Geometry: final body of the model. Coordinates: model frame, mm. A direction names the side the tool comes from. Round coordinates to 2 decimals unless told otherwise and drop trailing zeros. Write each loop counter-clockwise with the first axis right and the second up, starting at its lowest first coordinate (ties: lowest second). Pieces come first, ordered by that corner, then holes. Notation, with made-up numbers: (-30.75, -15) - (1.25, -15) arc R21 ccw to (1.25, 5) - close; hole circle Ø11 at (9.25, 38.25). An arc over 180 degrees is marked (long way). Use a Markdown table: item, result. Add a question column.
```python
from build123d import *

# Parameters (mm, degrees)
SKETCH1_W           = 37
SKETCH1_H           = 8
SKETCH1_R           = 1.75
BOSS_EXTRUDE1_DEPTH = 5
SKETCH2_W           = 4
SKETCH2_H           = 8
BOSS_EXTRUDE2_DEPTH = 12.5
SKETCH4_W           = 4
SKETCH4_H           = 7.5
BOSS_EXTRUDE3_DEPTH = 8
SKETCH3_R           = 1.75
CUT_EXTRUDE1_DEPTH  = 37.745748053
FILLET1_R           = 4
SKETCH6_R           = 1.6
BOSS_EXTRUDE5_DEPTH = 4


with BuildPart() as part:
    # Sketch1 → Boss-Extrude1 (new body)
    with BuildSketch(Plane.XY):
        Rectangle(SKETCH1_W, SKETCH1_H)
        with Locations((-15, 0)):
            Circle(SKETCH1_R, mode=Mode.SUBTRACT)
        with Locations(Location((15, 0, 0), (0, 0, 180))):
            Circle(SKETCH1_R, mode=Mode.SUBTRACT)
    extrude(amount=BOSS_EXTRUDE1_DEPTH)

    # Sketch2 → Boss-Extrude2 (add)
    with BuildSketch(Plane.XY.offset(5)):
        with Locations((-9.5, 0)):
            Rectangle(SKETCH2_W, SKETCH2_H)
        with Locations((9.5, 0)):
            Rectangle(SKETCH2_W, SKETCH2_H)
    extrude(amount=BOSS_EXTRUDE2_DEPTH)

    # Sketch4 → Boss-Extrude3 (add)
    with BuildSketch(Plane(origin=(0, 4, 0), x_dir=(1, 0, 0), z_dir=(0, 1, 0))):
        with Locations((-9.5, -13.75)):
            Rectangle(SKETCH4_W, SKETCH4_H)
        with Locations((9.5, -13.75)):
            Rectangle(SKETCH4_W, SKETCH4_H)
    extrude(amount=BOSS_EXTRUDE3_DEPTH)

    # Sketch3 → Cut-Extrude1 (cut, through all)
    with BuildSketch(Plane.ZY.offset(11.5)):
        with Locations(Location((13.75, 8.5, 0), (0, 0, 270))):
            Circle(SKETCH3_R)
    extrude(amount=-CUT_EXTRUDE1_DEPTH, mode=Mode.SUBTRACT)

    # Fillet1
    # the kernel refuses this fillet: 4 mm, written as the material it takes off along each edge
    with BuildSketch(Plane(origin=(2.5, 12, 10), x_dir=(0, -1, 0), z_dir=(-1, 0, 0))) as fillet1_piece_1:
        with BuildLine():
            CenterArc((FILLET1_R, FILLET1_R), FILLET1_R, 180, 90)
            Line((0, FILLET1_R), (0, 0))
            Line((0, 0), (FILLET1_R, 0))
        make_face()
    extrude(amount=24, mode=Mode.SUBTRACT)
    with BuildSketch(Plane(origin=(-2.5, 12, 10), x_dir=(0, -1, 0), z_dir=(1, 0, 0)), Plane(origin=(21.5, 12, 17.5), x_dir=(0, -1, 0), z_dir=(-1, 0, 0)), Plane(origin=(-21.5, 12, 17.5), x_dir=(0, 0, -1), z_dir=(1, 0, 0))) as fillet1_piece_2:
        with BuildLine():
            CenterArc((FILLET1_R, -FILLET1_R), FILLET1_R, 90, 90)
            Line((0, -FILLET1_R), (0, 0))
            Line((0, 0), (FILLET1_R, 0))
        make_face()
    extrude(amount=24, mode=Mode.SUBTRACT)

    # Sketch6 → Boss-Extrude5 (add)
    with BuildSketch(Plane.ZY.offset(11.5)):
        with BuildLine():
            Line((56.011251263, -29.401227517), (11.782401197, -4))
            Line((11.782401197, -4), (17.5, 1.941786969))
            Line((17.5, 1.941786969), (59.995440826, -22.463920148))
            ThreePointArc((59.995440826, -22.463920148), (61.471999729, -27.924668614), (56.011251263, -29.401227517))
        make_face()
        with Locations(Location((58.003346044, -25.932573832, 0), (0, 0, 270))):
            Circle(SKETCH6_R, mode=Mode.SUBTRACT)
    extrude(amount=-BOSS_EXTRUDE5_DEPTH)


solid = part.part
```
1) Section A-A, the plane x = -15. Return the cut outline in (y, z), then the cut area to 3 significant figures.
2) Set-up query: faces 1 (the flat face through (9, 6, 10)), 2 (the flat face through (7.5, 2, 11)), 3 (the flat face through (-15, 2, 5)), 4 (the flat face through (-10, 5, 17.5)). Return all of +Z, -Z, +X, -X, +Y, -Y with unobstructed straight access to the full face (end or side cutting, diameter ignored); none if empty.
3) Pin query (flat end, axial travel): P1, Ø6, axis at x = -11.5, z = 37.5, coming from the +Y side; P2, Ø4.5, axis at x = -8.5, y = 4, coming from the +Z side; P3, Ø21, axis at y = -12.5, z = 21, coming from the -X side. Return the tip coordinate at first contact, or that it passes through.
4) Section C-C, the plane y = 0. Return the cut outline in (x, z), then the cut area to 3 significant figures.
5) Section D-D, the plane x = 1. Return the cut outline in (y, z).
6) Section B-B, the plane z = 9. Return the cut outline in (x, y).
7) Draft query along Z for faces 5 (the flat face through (-0.3, -4, 4.7)), 6 (the cylindrical face through (-9.528, -27.848, 61.515)), 7 (the cylindrical face through (-9.53, -25.72, 59.59)). Return one class per face: released by +Z, released by -Z, zero draft, split by the parting line, or undercut.
8) Material intervals for L1, parallel to Y at x = 15, z = 1.95; L2, parallel to Z at x = -12, y = -2; L3, parallel to X at y = -17.5, z = 38.5, sorted ascending. Write a range as from..to.
Output values:
| question | item | result |
|---|---|---|
| 1 | outline | (-4, 0) - (-1.75, 0) - (-1.75, 5) - (-4, 5) - close; (1.75, 0) - (4, 0) - (4, 5) - (1.75, 5) - close |
| 1 | area | 22.5 mm^2 |
| 2 | face 1 | -Z, +X, -X, +Y |
| 2 | face 2 | +Z, +Y, -Y |
| 2 | face 3 | +Z, -X, +Y, -Y |
| 2 | face 4 | +Z, +X, -X, +Y |
| 3 | P1 | stops at y = -7.82 |
| 3 | P2 | stops at z = 17.83 |
| 3 | P3 | stops at x = -11.5 |
| 4 | outline | (-18.5, 0) - (-16.75, 0) - (-16.75, 5) - (-18.5, 5) - close; (-13.25, 0) - (13.25, 0) - (13.25, 5) - (11.5, 5) - (11.5, 17.5) - (7.5, 17.5) - (7.5, 5) - (-7.5, 5) - (-7.5, 20.88) - (-11.5, 20.88) - (-11.5, 5) - (-13.25, 5) - close; (16.75, 0) - (18.5, 0) - (18.5, 5) - (16.75, 5) - close |
| 4 | area | 264 mm^2 |
| 5 | outline | (-4, 0) - (4, 0) - (4, 5) - (-4, 5) - close |
| 6 | outline | (-11.5, -4) - (-7.5, -4) - (-7.5, 4) - (-11.5, 4) - close; (7.5, -4) - (11.5, -4) - (11.5, 4) - (7.5, 4) - close |
| 7 | face 5 | zero draft |
| 7 | face 6 | split by the parting line |
| 7 | face 7 | undercut |
| 8 | L1 | y = -4..-1.75, 1.75..4 |
| 8 | L2 | z = 0..5 |
| 8 | L3 | x = -11.5..-7.5 |
